Design review of the part built by this model. Coordinates are the model's own, in mm. Face numbers are marked on the shaded views. Give positions to 0.01 mm unless a question says otherwise; leave off trailing zeros. Loops run counter-clockwise (first coordinate to the right, second up) from the corner with the lowest first, then second, coordinate; pieces in that order, holes last. Notation, with made-up numbers: (24, -7) -> (78, -7) arc R19 cw to (78, 19) -> close; hole circle Ø11 at (-4.5, -32.75). An arc over 180 degrees is marked (long way). Answer as CSV lines item,"result".
Autodesk Inventor part; units mm, degrees
ref_plane "YZ Plane" through (0, 0, 0) normal (1, 0, 0) x (0, 1, 0)
ref_plane "XZ Plane" through (0, 0, 0) normal (0, 1, 0) x (-1, 0, 0)
ref_plane "XY Plane" through (0, 0, 0) normal (0, 0, 1) x (1, 0, 0)
sketch "Sketch1" plane through (0, 0, 0) normal (0, 1, 0) x (-1, 0, 0)
  line L0 (38.1, 50.8) -> (-38.1, 50.8)
  line L1 (-38.1, 50.8) -> (-38.1, -50.8)
  line L2 (-38.1, -50.8) -> (38.1, -50.8)
  line L3 (38.1, -50.8) -> (38.1, 50.8)
  point P0 (0, 0)
  dimension "d0" = 101.6
  dimension "d1" = 76.2
  dimension "d2" = 38.1
  dimension "d3" = 50.8
extrude "Extrusion1" add sketch "Sketch1" along normal blind 50.8
sketch "Sketch2" plane through (-38.1, 0, 50.8) normal (0, 0, 1) x (1, 0, 0)
  line L0 (76.2, 50.8) -> (0, 50.8)
  line L1 (76.2, 0) -> (0, 0)
  line L2 (0, 50.8) -> (3.175, 50.8)
  line L3 (3.175, 50.8) -> (3.175, 0)
  line L4 (0, 0) -> (0, 50.8)
  line L5 (76.2, 0) -> (76.2, 50.8)
  line L6 (0, 50.8) -> (76.2, 50.8)
  line L7 (76.2, 50.8) -> (76.2, 47.625)
  line L8 (0, 47.625) -> (0, 50.8)
  line L9 (76.2, 50.8) -> (73.025, 50.8)
  line L10 (73.025, 50.8) -> (73.025, 0)
  line L11 (76.2, 0) -> (76.2, 50.8)
  line L12 (3.175, 15.875) -> (6.35, 15.875)
  line L13 (6.35, 15.875) -> (6.35, 19.05)
  line L14 (6.35, 19.05) -> (3.175, 19.05)
  line L15 (3.175, 19.05) -> (3.175, 15.875)
  line L16 (3.175, 25.4) -> (6.35, 25.4)
  line L17 (6.35, 25.4) -> (6.35, 28.575)
  line L18 (6.35, 28.575) -> (3.175, 28.575)
  line L19 (3.175, 28.575) -> (3.175, 25.4)
  line L20 (38.1, 47.625) -> (38.1, 0)
  line L21 (73.025, 15.875) -> (69.85, 15.875)
  line L22 (69.85, 15.875) -> (69.85, 19.05)
  line L23 (69.85, 19.05) -> (73.025, 19.05)
  line L24 (73.025, 25.4) -> (69.85, 25.4)
  line L25 (69.85, 25.4) -> (69.85, 28.575)
  line L26 (69.85, 28.575) -> (73.025, 28.575)
  line L27 (3.175, 50.8) -> (6.35, 50.8)
  line L28 (6.35, 50.8) -> (6.35, 47.625)
  line L29 (6.35, 47.625) -> (3.175, 47.625)
  line L30 (3.175, 47.625) -> (3.175, 50.8)
  line L31 (73.025, 50.8) -> (69.85, 50.8)
  line L32 (69.85, 50.8) -> (69.85, 47.625)
  line L33 (69.85, 47.625) -> (73.025, 47.625)
  line L34 (73.025, 47.625) -> (73.025, 50.8)
  line L35 (0, 0) -> (76.2, 0)
  line L36 (76.2, 0) -> (76.2, 3.175)
  line L37 (76.2, 3.175) -> (0, 3.175)
  line L38 (0, 3.175) -> (0, 0)
  point P0 (3.175, 3.175)
  point P1 (73.025, 3.175)
  point P2 (6.35, 50.8)
  point P3 (3.175, 47.625)
  point P4 (3.175, 28.575)
  point P5 (3.175, 19.05)
  dimension "d6" = 3.175
  dimension "d8" = 3.175
  dimension "d11" = 3.175
  dimension "d12" = 3.175
  dimension "d13" = 3.175
  dimension "d15" = 6.35
  dimension "d16" = 3.175
  dimension "d17" = 12.7
  dimension "d18" = 0
extrude "Extrusion2" cut sketch "Sketch2" against normal blind 98.425 contours L32 L33 L10 L26 L25 L24 L23 L22 L21 L37 L3 L12 L13 L14 L16 L17 L18 L29 L28 L0
sketch "Sketch3" plane through (38.1, 0, -50.8) normal (0, 0, -1) x (-1, 0, 0)
  line L0 (0, 50.8) -> (76.2, 50.8)
  line L1 (38.1, 0) -> (38.1, 50.8) construction
  line L2 (29.21, 50.8) -> (36.83, 50.8)
  line L3 (36.83, 50.8) -> (36.83, 31.75)
  line L4 (29.21, 31.75) -> (29.21, 50.8)
  line L5 (26.67, 50.8) -> (19.05, 50.8)
  line L6 (19.05, 50.8) -> (19.05, 31.75)
  line L7 (26.67, 31.75) -> (26.67, 50.8)
  line L8 (33.02, 31.75) -> (33.02, 50.8) construction
  line L9 (22.86, 31.75) -> (22.86, 50.8) construction
  line L10 (16.51, 50.8) -> (8.89, 50.8)
  line L11 (8.89, 50.8) -> (8.89, 31.75)
  line L12 (16.51, 31.75) -> (16.51, 50.8)
  line L13 (12.7, 31.75) -> (12.7, 50.8) construction
  arc A0 (8.89, 31.75) -> (16.51, 31.75) centre (12.7, 31.75) ccw
  arc A1 (19.05, 31.75) -> (26.67, 31.75) centre (22.86, 31.75) ccw
  arc A2 (29.21, 31.75) -> (36.83, 31.75) centre (33.02, 31.75) ccw
  line L14 (8.89, 31.75) -> (36.83, 31.75) construction
  line L15 (46.99, 50.8) -> (39.37, 50.8)
  line L16 (39.37, 50.8) -> (39.37, 31.75)
  line L17 (46.99, 31.75) -> (46.99, 50.8)
  line L18 (49.53, 50.8) -> (57.15, 50.8)
  line L19 (57.15, 50.8) -> (57.15, 31.75)
  line L20 (49.53, 31.75) -> (49.53, 50.8)
  line L21 (43.18, 31.75) -> (43.18, 50.8) construction
  line L22 (53.34, 31.75) -> (53.34, 50.8) construction
  line L23 (59.69, 50.8) -> (67.31, 50.8)
  line L24 (67.31, 50.8) -> (67.31, 31.75)
  line L25 (59.69, 31.75) -> (59.69, 50.8)
  line L26 (63.5, 31.75) -> (63.5, 50.8) construction
  arc A3 (59.69, 31.75) -> (67.31, 31.75) centre (63.5, 31.75) ccw
  arc A4 (49.53, 31.75) -> (57.15, 31.75) centre (53.34, 31.75) ccw
  arc A5 (39.37, 31.75) -> (46.99, 31.75) centre (43.18, 31.75) ccw
  line L27 (67.31, 31.75) -> (39.37, 31.75) construction
  point P0 (19.05, 50.8)
  point P1 (8.89, 50.8)
  dimension "d21" = 10.16
  dimension "d22" = 5.08
  dimension "d24" = 7.62
  dimension "d25" = 7.62
  dimension "d26" = 10.16
  dimension "d27" = 7.62
  dimension "d28" = 19.05
extrude "Extrusion3" cut sketch "Sketch3" against normal blind 3.175
sketch "Sketch4" plane through (38.1, 0, 50.8) normal (1, 0, 0) x (0, 0, -1)
  line L0 (50.8, 0) -> (50.8, 50.8) construction
  line L1 (0, 50.8) -> (101.6, 50.8)
  line L2 (44.45, 50.8) -> (57.15, 50.8)
  line L3 (57.15, 50.8) -> (57.15, 47.625)
  line L4 (57.15, 47.625) -> (44.45, 47.625)
  line L5 (44.45, 47.625) -> (44.45, 50.8)
  point P0 (57.15, 50.8)
  dimension "d31" = 3.175
  dimension "d32" = 12.7
  dimension "d33" = 6.35
extrude "Extrusion4" add sketch "Sketch4" along normal blind 12.7
sketch "Sketch5" plane through (-38.1, 0, -50.8) normal (-1, 0, 0) x (0, 0, 1)
  line L0 (50.8, 0) -> (50.8, 50.8) construction
  line L1 (44.45, 50.8) -> (57.15, 50.8)
  line L2 (57.15, 50.8) -> (57.15, 47.625)
  line L3 (57.15, 47.625) -> (44.45, 47.625)
  line L4 (44.45, 47.625) -> (44.45, 50.8)
  dimension "d36" = 3.175
  dimension "d37" = 12.7
  dimension "d38" = 6.35
extrude "Extrusion5" add sketch "Sketch5" along normal blind 12.7
sketch "Sketch6" plane through (-38.1, 47.625, -6.35) normal (0, -1, 0) x (1, 0, 0)
  line L0 (0, 0) -> (-12.7, 0)
  line L1 (-6.35, 0) -> (-6.35, 12.7) construction
  line L2 (0, 12.7) -> (-12.7, 12.7)
  circle A0 centre (-6.35, 6.35) radius 3.81
  point P0 (38.1, 6.35)
  dimension "d41" = 7.62
extrude "Extrusion6" cut sketch "Sketch6" against normal blind 12.7
sketch "Sketch7" plane through (38.1, 47.625, -6.35) normal (0, -1, 0) x (1, 0, 0)
  line L0 (0, 12.7) -> (12.7, 12.7)
  line L1 (6.35, 12.7) -> (6.35, 0) construction
  line L2 (0, 0) -> (12.7, 0)
  circle A0 centre (6.35, 6.35) radius 3.81
  point P0 (-38.1, 6.35)
  dimension "d44" = 7.62
extrude "Extrusion7" cut sketch "Sketch7" against normal blind 12.7
equation "\"d8\" = d6"
equation "\"d11\" = d6"
equation "\"d12\" = d6"
equation "\"d13\" = d6"
equation "\"d33\" = 0.5 * d32"
equation "\"d38\" = 0.5 * d37"
properties part number "main"
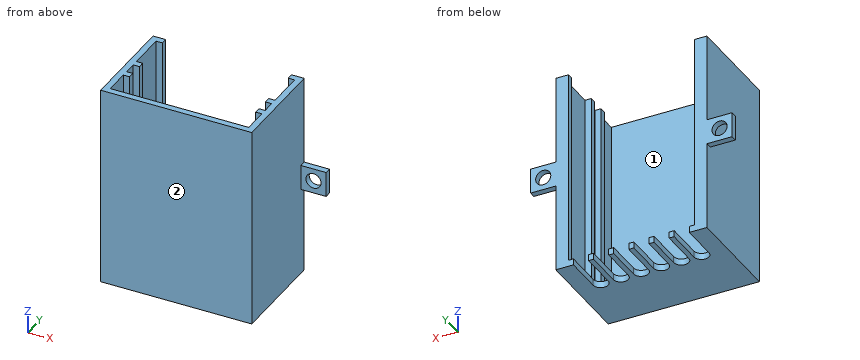
Q1. To check wall thickness, follow probe 1 along Z at (x, y) = (44.45, 50.1); probe 2 along X at (y, z) = (14.5, -10) (3 decimals); probe 3 along X at (y, z) = (49.5, -44). State the ranges of each line that lie inside material, in increasing order. Write a range as from..to.
Filled sheet:
probe 1,"z = -6.35..-3.81, 3.81..6.35"
probe 2,"x = -38.1..-34.925, 34.925..38.1"
probe 3,"x = -38.1..-31.75, 31.75..38.1"
Q2. We need section A-A, the plane x = -44.45. State the section outline as (y, z) points (3 decimals).
Filled sheet:
outline,"(47.625, -6.35) -> (50.8, -6.35) -> (50.8, -3.81) -> (47.625, -3.81) -> close; (47.625, 3.81) -> (50.8, 3.81) -> (50.8, 6.35) -> (47.625, 6.35) -> close"
Q3. We need section C-C, the plane y = 38. State how many separate pieces and enclosed holes the cut face has, and give its area (3 significant figures).
Filled sheet:
separate pieces,"7"
enclosed holes,"0"
area,"722 mm^2"
Q4. We need section D-D, the plane x = 5.08. State the section outline as (y, z) points (3 decimals).
Filled sheet:
outline,"(0, -50.8) -> (27.94, -50.8) -> (27.94, -47.625) -> (3.175, -47.625) -> (3.175, 50.8) -> (0, 50.8) -> close"
Q5. Clearance check with flat-ended pins moving along their axes: pin 1 Ø6 at (y, z) = (10, 27) entering from +X; pin 2 Ø1.6 at (y, z) = (37.5, -49) entering from -X; pin 3 Ø6 at (x, z) = (-44.45, 0) entering from -Y. State where each tip first meets the part, or that it passes through.
Filled sheet:
pin 1,"stops at x = 38.1"
pin 2,"stops at x = -38.1"
pin 3,"passes through"
Q6. The part is to be moulded in two halves that separate along X. For the marked faces 1 and 2, say which applies: pulls with the +X half, pulls with the -X half, needs draft (parallel to the pull), parting line crosses it, or undercut.
Filled sheet:
face 1,"undercut"
face 2,"needs draft"
Q7. We need section B-B, the plane z = -17. State the section outline as (x, y) points (3 decimals).
Filled sheet:
outline,"(-38.1, 0) -> (38.1, 0) -> (38.1, 50.8) -> (31.75, 50.8) -> (31.75, 47.625) -> (34.925, 47.625) -> (34.925, 28.575) -> (31.75, 28.575) -> (31.75, 25.4) -> (34.925, 25.4) -> (34.925, 19.05) -> (31.75, 19.05) -> (31.75, 15.875) -> (34.925, 15.875) -> (34.925, 3.175) -> (-34.925, 3.175) -> (-34.925, 15.875) -> (-31.75, 15.875) -> (-31.75, 19.05) -> (-34.925, 19.05) -> (-34.925, 25.4) -> (-31.75, 25.4) -> (-31.75, 28.575) -> (-34.925, 28.575) -> (-34.925, 47.625) -> (-31.75, 47.625) -> (-31.75, 50.8) -> (-38.1, 50.8) -> close"
